Model file for the job. Use its own axes, mm. Face numbers are marked on the shaded views. Round coordinates to 2 decimals unless told otherwise and drop trailing zeros. Order: outer loops, then holes, each group sorted by start corner. A loop starts at its lowest first (then second) coordinate and runs counter-clockwise, first axis right, second up. Notation, with made-up numbers: (86.25, -19.75) - (92.25, -19.75) arc R31 ccw to (92.25, 4.25) - close; hole circle Ø2 at (88, -30.75). An arc over 180 degrees is marked (long way). Write item = value, one per line.
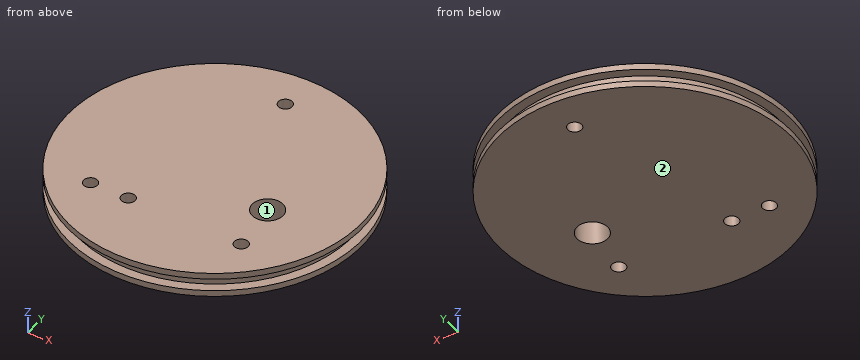
```python
from build123d import *

# Parameters (mm, degrees)
BOSS_EXTRUDE1_DEPTH      = 8
BOSS_EXTRUDE1_DEPTH_BACK = 8
SKETCH2_R                = 95
CUT_EXTRUDE1_DEPTH       = 4
CUT_EXTRUDE1_DEPTH_BACK  = 4
SKETCH2_5_R              = 95
SKETCH2_5_R_2            = 89
SKETCH7_R                = 4.5
CUT_EXTRUDE2_DEPTH       = 167
CUT_EXTRUDE4_DEPTH       = 112
CUT_EXTRUDE4_DEPTH_BACK  = 60
SKETCH10_R               = 4.5
SKETCH11_R               = 10
CUT_EXTRUDE5_DEPTH       = 60


with BuildPart() as part:
    # Sketch2 → Boss-Extrude1 (new, two sides: drawn at the far end of the back side and taken through both)
    with BuildSketch(Plane.XY.offset(-BOSS_EXTRUDE1_DEPTH_BACK)):
        Circle(SKETCH2_R)
    extrude(amount=BOSS_EXTRUDE1_DEPTH + BOSS_EXTRUDE1_DEPTH_BACK)

    # Sketch2_5 → Cut-Extrude1 (cut, two sides: drawn at the far end of the back side and taken through both)
    with BuildSketch(Plane.XY.offset(-CUT_EXTRUDE1_DEPTH_BACK)):
        Circle(SKETCH2_5_R)
        Circle(SKETCH2_5_R_2, mode=Mode.SUBTRACT)
    extrude(amount=CUT_EXTRUDE1_DEPTH + CUT_EXTRUDE1_DEPTH_BACK, mode=Mode.SUBTRACT)

    # Sketch7 → Cut-Extrude2 (cut)
    with BuildSketch(Plane.XY.offset(8)):
        with Locations((-50, -48.75)):
            Circle(SKETCH7_R)
        with Locations((50, -48.75)):
            Circle(SKETCH7_R)
        with Locations((-25, -48.75)):
            Circle(SKETCH7_R)
    extrude(amount=-CUT_EXTRUDE2_DEPTH, mode=Mode.SUBTRACT)

    # Sketch10 → Cut-Extrude4 (cut, two sides: drawn at the far end of the back side and taken through both)
    with BuildSketch(Plane(origin=(0, 0, -8), x_dir=(-1, 0, 0), z_dir=(0, 0, -1)).offset(-CUT_EXTRUDE4_DEPTH_BACK)):
        with Locations(Location((0, 70, 0), (0, 0, 180))):
            Circle(SKETCH10_R)
    extrude(amount=CUT_EXTRUDE4_DEPTH + CUT_EXTRUDE4_DEPTH_BACK, mode=Mode.SUBTRACT)

    # Sketch11 → Cut-Extrude5 (cut)
    with BuildSketch(Plane(origin=(0, 0, -8), x_dir=(-1, 0, 0), z_dir=(0, 0, -1))):
        with Locations((-45, -15)):
            Circle(SKETCH11_R)
    extrude(amount=-CUT_EXTRUDE5_DEPTH, mode=Mode.SUBTRACT)


solid = part.part
```
1) Cut at A-A (x = 0). Write the cut outline in (y, z), and give its area (3 significant figures).
Conclusion:
outline = (-95, -8) - (65.5, -8) - (65.5, 8) - (-95, 8) - (-95, 4) - (-89, 4) - (-89, -4) - (-95, -4) - close; (74.5, -8) - (95, -8) - (95, -4) - (89, -4) - (89, 4) - (95, 4) - (95, 8) - (74.5, 8) - close
area = 2,800 mm^2
2) Wall check: line 1 along Y through (x, z) = (0, 2); line 2 along Z through (x, y) = (78.5, 47); line 3 along Y through (x, z) = (45, -1.5). Give the ranges that are in metal, low to high.
Conclusion:
line_1 = -89 to 65.5, 74.5 to 89
line_2 = -8 to -4, 4 to 8
line_3 = -76.79 to -25, -5 to 76.79
3) Cut at C-C (x = 50). Write the cut outline in (y, z), and give its area (3 significant figures).
Conclusion:
outline = (-80.78, -8) - (-53.25, -8) - (-53.25, 8) - (-80.78, 8) - (-80.78, 4) - (-73.63, 4) - (-73.63, -4) - (-80.78, -4) - close; (-44.25, -8) - (-23.66, -8) - (-23.66, 8) - (-44.25, 8) - close; (-6.34, -8) - (80.78, -8) - (80.78, -4) - (73.63, -4) - (73.63, 4) - (80.78, 4) - (80.78, 8) - (-6.34, 8) - close
area = 2,050 mm^2
4) Mould opens along Y. For the marked faces 1 and 2 say: +Y half, -Y half, draft (parallel to the pull), parting line (faces both ways), or undercut.
Conclusion:
face_1 = undercut
face_2 = draft
5) Cut at D-D (y = -48.75). Write the cut outline in (x, z), and give its area (3 significant figures).
Conclusion:
outline = (-81.54, -8) - (-54.5, -8) - (-54.5, 8) - (-81.54, 8) - (-81.54, 4) - (-74.46, 4) - (-74.46, -4) - (-81.54, -4) - close; (-45.5, -8) - (-29.5, -8) - (-29.5, 8) - (-45.5, 8) - close; (-20.5, -8) - (45.5, -8) - (45.5, 8) - (-20.5, 8) - close; (54.5, -8) - (81.54, -8) - (81.54, -4) - (74.46, -4) - (74.46, 4) - (81.54, 4) - (81.54, 8) - (54.5, 8) - close
area = 2,060 mm^2
6) Flat gauge pins, fed straight in: pin 1 Ø4 at (x, z) = (-25.5, 1.5) entering from +Y; pin 2 Ø6 at (x, z) = (-74, 1.5) entering from +Y; pin 3 Ø1.5 at (y, z) = (76, -5.5) entering from -X. Where does each tip first touch, or does it go through?
Conclusion:
pin_1 = 85.84
pin_2 = 61.58
pin_3 = -57.99
7) Cut at B-B (y = 0). Write the cut outline in (x, z), and give its area (3 significant figures).
Conclusion:
outline = (-95, -8) - (95, -8) - (95, -4) - (89, -4) - (89, 4) - (95, 4) - (95, 8) - (-95, 8) - (-95, 4) - (-89, 4) - (-89, -4) - (-95, -4) - close
area = 2,940 mm^2
